Geometry: final body of the model. Coordinates: model frame, mm. A direction names the side the tool comes from. Round coordinates to 2 decimals unless told otherwise and drop trailing zeros. Loops run counter-clockwise (first coordinate to the right, second up) from the corner with the lowest first, then second, coordinate; pieces in that order, holes last. Notation, with made-up numbers: (2, -33) - (50, -33) arc R26 cw to (50, -16) - close; hole circle Ø9 at (-3.5, 67). An arc over 180 degrees is marked (long way). Return JSON: item names as keys, results as strings. Group by question number.
1. Section D-D on z = 12. Return loops of the section in (x, y).
2. Section B-B on z = 88. Return loops of the section in (x, y), and give its area (3 significant figures).
3. Set-up query: faces 1 (the face through (-383, 212, 127)), 2 (the face through (-386, 203.2, 63)). Return all of +Z, -Z, +X, -X, +Y, -Y with unobstructed straight access to the full face (end or side cutting, diameter ignored); none if empty.
4. First-contact query: pin 1 Ø8 at (y, z) = (187.5, 19) entering from +X. Flat tip, straight axial feed; report the tip coordinate or a pass-through.
5. Draft query along X for faces 3 (the face through (68.96, 271.76, 64.03)), 4 (the face through (-830.56, 272.16, 64.03)), 5 (the face through (-375, 279.4, 63)), 6 (the face through (0, 103, 63)). Return one class per face: +X half, -X half, draft (parallel to the pull), parting line (faces both ways), or undercut.
6. Material intervals for probe 1 along X at (y, z) = (38, 87); probe 2 along Y at (x, z) = (-597, 57); probe 3 along X at (y, z) = (159, 106), sorted ascending.
7. Section C-C on x = -582. Return loops of the section in (y, z), and give its area (3 significant figures).
8. Section A-A on y = 101. Return loops of the section in (x, z).
Autodesk Inventor part; units mm, degrees
ref_plane "YZ Plane" through (0, 0, 0) normal (1, 0, 0) x (0, 1, 0)
ref_plane "XZ Plane" through (0, 0, 0) normal (0, 1, 0) x (-1, 0, 0)
ref_plane "XY Plane" through (0, 0, 0) normal (0, 0, 1) x (1, 0, 0)
sketch "Sketch1" plane through (0, 0, 0) normal (0, 0, 1) x (1, 0, 0)
  line L0 (0, 0) -> (76.2, 0)
  line L1 (76.2, 0) -> (76.2, 279.4)
  line L2 (76.2, 279.4) -> (0, 279.4)
  line L3 (0, 279.4) -> (0, 0)
  line L4 (0, 279.4) -> (-838.2, 279.4)
  line L5 (-838.2, 279.4) -> (-838.2, 203.2)
  line L6 (-838.2, 203.2) -> (0, 203.2)
  line L7 (0, 203.2) -> (0, 279.4)
  line L8 (-838.2, 203.2) -> (-762, 203.2)
  line L9 (-762, 203.2) -> (-762, 0)
  line L10 (-762, 0) -> (-838.2, 0)
  line L11 (-838.2, 0) -> (-838.2, 203.2)
  dimension "d0" = 76.2
  dimension "d1" = 279.4
  dimension "d2" = 838.2
  dimension "d3" = 76.2
  dimension "d4" = 76.2
  dimension "d5" = 203.2
extrude "Extrusion1" add sketch "Sketch1" along normal blind 127
sketch "Sketch2" plane through (-838.2, 279.4, 0) normal (0, 1, 0) x (1, 0, 0)
  line L0 (642.6606, -111.4085) -> (325.9156, -111.4085) construction
  line L1 (325.9156, -111.4085) -> (325.9156, -9.0111) construction
  line L2 (325.9156, -9.0111) -> (642.6606, -9.0111) construction
  line L3 (642.6606, -9.0111) -> (642.6606, -111.4085) construction
  point P0 (838.2, 0)
fillet "Fillet1" radius 25.4 8 edges at (-381, 279.4, 127) (-381, 279.4, 0) (76.2, 139.7, 127) (76.2, 139.7, 0) (76.2, 279.4, 63.5) (-838.2, 279.4, 63.5) (-838.2, 139.7, 127) (-838.2, 139.7, 0)
properties part number "bumper" material "Canvas, Blue Stripe"
Taken from the geometry:
{
 "1": {"outline": "(-834.38, 0) - (-762, 0) - (-762, 203.2) - (0, 203.2) - (0, 0) - (72.38, 0) - (72.38, 254) arc R21.58 ccw to (50.8, 275.58) - (-812.8, 275.58) arc R21.58 ccw to (-834.38, 254) - close"},
 "2": {"outline": "(-838.2, 0) - (-762, 0) - (-762, 203.2) - (0, 203.2) - (0, 0) - (76.2, 0) - (76.2, 254) arc R25.4 ccw to (50.8, 279.4) - (-812.8, 279.4) arc R25.4 ccw to (-838.2, 254) - close", "area": "100,000 mm2"},
 "3": {"face 1": "+Z, +X, -X, +Y, -Y", "face 2": "+Z, -Z, -Y"},
 "4": {"pin 1": "x = 76.09"},
 "5": {"face 3": "+X half", "face 4": "-X half", "face 5": "draft", "face 6": "undercut"},
 "6": {"probe 1": "-838.2 to -762, 0 to 76.2", "probe 2": "203.2 to 279.4", "probe 3": "-837.82 to -762, 0 to 75.82"},
 "7": {"outline": "(203.2, 0) - (254, 0) arc R25.4 ccw to (279.4, 25.4) - (279.4, 101.6) arc R25.4 ccw to (254, 127) - (203.2, 127) - close", "area": "9,400 mm2"},
 "8": {"outline": "(-838.2, 25.4) arc R25.4 ccw to (-812.8, 0) - (-762, 0) - (-762, 127) - (-812.8, 127) arc R25.4 ccw to (-838.2, 101.6) - close; (0, 0) - (50.8, 0) arc R25.4 ccw to (76.2, 25.4) - (76.2, 101.6) arc R25.4 ccw to (50.8, 127) - (0, 127) - close"}
}
